Source: CAD feature listing. Evaluate the final solid. Frame: model axes, mm. Coordinates: 2 decimals unless noted, no trailing zeros. Order: outer loops, then holes, each group sorted by start corner. A loop starts at its lowest first (then second) coordinate and runs counter-clockwise, first axis right, second up.
Autodesk Inventor part; units mm, degrees
ref_plane "YZ Plane" through (0, 0, 0) normal (1, 0, 0) x (0, 1, 0)
ref_plane "XZ Plane" through (0, 0, 0) normal (0, 1, 0) x (-1, 0, 0)
ref_plane "XY Plane" through (0, 0, 0) normal (0, 0, 1) x (1, 0, 0)
sketch "Sketch1" plane through (0, 0, 0) normal (0, 0, 1) x (1, 0, 0)
  line L0 (-1.1274, 1.6306) -> (0.8726, 1.6306)
  line L1 (0.8726, 1.6306) -> (0.8726, -19.3694)
  line L2 (0.8726, -19.3694) -> (-1.1274, -19.3694)
  line L3 (-1.1274, -19.3694) -> (-1.1274, 1.6306)
  point P0 (0, 0)
  dimension "d0" = 2
  dimension "d1" = 21
extrude "Extrusion1" add sketch "Sketch1" along normal blind 83
sketch "Sketch2" plane through (0.8726, -19.3694, 0) normal (1, 0, 0) x (0, 0, -1)
  circle A0 centre (-23.0575, 8.9801) radius 2.5
  circle A1 centre (-23.0575, 8.9801) radius 2.5
  circle A2 centre (-23.0575, 8.9801) radius 2.5
  circle A3 centre (-44.0219, 8.9592) radius 2.5
  circle A4 centre (-44.0219, 8.9592) radius 2.5
  circle A5 centre (-44.0219, 8.9592) radius 2.5
  circle A6 centre (-44.0219, 8.9592) radius 2.5
  circle A7 centre (-44.0219, 8.9592) radius 2.5
  circle A8 centre (-70.0331, 8.9359) radius 2.5
  point P0 (0, 19.3694)
extrude "Extrusion2" cut sketch "Sketch2" against normal blind 10
properties part number "Gear wall motor side"
1. Material intervals for line 1 along Z through (x, y) = (-0.4, -10); line 2 along Z through (x, y) = (-0.75, -8.25); line 3 along Y through (x, z) = (-0.65, 70.5), sorted ascending.
2. Section query A-A, the plane z = 71. Output: boundary loops of the cut face in (x, y).
3. Section query B-B, the plane y = -12. Output: boundary loops of the cut face in (x, z), plus the area to 3 significant figures.
4. Section query C-C, the plane x = 0.55. Output: boundary loops of the cut face in (y, z), plus the area to 3 significant figures.
5. Draft query along Z for faces 1 (the flat face through (0, 1.631, 41)), 2 (the cylindrical face through (-0.11, -9.68, 67.65)), 3 (the flat face through (0, -9, 83)). Return one class per face: +Z half, -Z half, draft (parallel to the pull), parting line (faces both ways), or undercut.
Answer key:
1. line 1: z = 0 to 20.59, 25.53 to 41.56, 46.49 to 67.57, 72.5 to 83
1. line 2: z = 0 to 21.76, 24.35 to 42.76, 45.28 to 68.82, 71.25 to 83
1. line 3: y = -19.37 to -12.89, -7.98 to 1.63
2. outline: (-1.13, -19.37) - (0.87, -19.37) - (0.87, -12.74) - (-1.13, -12.74) - close; (-1.13, -8.13) - (0.87, -8.13) - (0.87, 1.63) - (-1.13, 1.63) - close
3. outline: (-1.13, 0) - (0.87, 0) - (0.87, 21.15) - (-1.13, 21.15) - close; (-1.13, 24.97) - (0.87, 24.97) - (0.87, 42.09) - (-1.13, 42.09) - close; (-1.13, 45.95) - (0.87, 45.95) - (0.87, 68.08) - (-1.13, 68.08) - close; (-1.13, 71.98) - (0.87, 71.98) - (0.87, 83) - (-1.13, 83) - close
3. area: 143 mm2
4. outline: (-19.37, 0) - (1.63, 0) - (1.63, 83) - (-19.37, 83) - close; hole circle Ø5 at (-10.43, 70.03); hole circle Ø5 at (-10.41, 44.02); hole circle Ø5 at (-10.39, 23.06)
4. area: 1,680 mm2
5. face 1: draft
5. face 2: undercut
5. face 3: +Z half
